from build123d import *

# Parameters (mm, degrees)
SKETCH1_R           = 10.5
SKETCH1_R_2         = 8
BOSS_EXTRUDE1_DEPTH = 3


with BuildPart() as part:
    # Sketch1 → Boss-Extrude1 (new body)
    # profile 1 of 4: a face of its own
    with BuildSketch(Plane.XY):
        Circle(SKETCH1_R)
        Circle(SKETCH1_R_2, mode=Mode.SUBTRACT)
    # profile 2 of 4: a face of its own
    with BuildSketch(Plane.XY):
        with BuildLine():
            ThreePointArc((1, 7.937253933), (0, 8), (-1, 7.937253933))
            Line((-1, 7.937253933), (-1, 5.937253933))
            ThreePointArc((-1, 5.937253933), (0, 6.020879028), (1, 5.937253933))
            Line((1, 5.937253933), (1, 7.937253933))
        make_face()
    # profile 3 of 4: a face of its own
    with BuildSketch(Plane.XY):
        with BuildLine():
            ThreePointArc((6.373863542, -4.83465237), (6.92820323, -4), (7.373863542, -3.102601563))
            Line((7.373863542, -3.102601563), (5.641812735, -2.102601563))
            ThreePointArc((5.641812735, -2.102601563), (5.214234191, -3.010439514), (4.641812735, -3.83465237))
            Line((4.641812735, -3.83465237), (6.373863542, -4.83465237))
        make_face()
    # profile 4 of 4: a face of its own
    with BuildSketch(Plane.XY):
        with BuildLine():
            Line((-5.641812735, -2.102601563), (-7.373863542, -3.102601563))
            ThreePointArc((-7.373863542, -3.102601563), (-6.92820323, -4), (-6.373863542, -4.83465237))
            Line((-6.373863542, -4.83465237), (-4.641812735, -3.83465237))
            ThreePointArc((-4.641812735, -3.83465237), (-5.214234191, -3.010439514), (-5.641812735, -2.102601563))
        make_face()
    extrude(amount=BOSS_EXTRUDE1_DEPTH)


solid = part.part
Verification items for the finished model (mm, model axes). A direction names the side the tool comes from. Give positions to 0.01 mm unless a question says otherwise; leave off trailing zeros. Write each loop counter-clockwise with the first axis right and the second up, starting at its lowest first coordinate (ties: lowest second). Pieces come first, ordered by that corner, then holes. Notation, with made-up numbers: M 31.5,87.25 L 65.5,87.25 A13 ccw 65.5,103.25 Z; hole C 33.5,14 d1. An arc over 180 degrees is marked long. Write item = value, one per line.
(1) Sectioned sample at D-D (x = 9). Record the cut outline in (y, z).
Found:
outline = M -5.41,0 L 5.41,0 L 5.41,3 L -5.41,3 Z
(2) Sectioned sample at B-B (x = 0). Record the cut outline in (y, z).
Found:
outline = M -10.5,0 L -8,0 L -8,3 L -10.5,3 Z; M 6.02,0 L 10.5,0 L 10.5,3 L 6.02,3 Z
(3) Material ranges on line 1 (X direction, y = 0.25, z = 0.7); line 2 (X direction, y = 6.75, z = 2.4); line 3 (Y direction, x = -6.25, z = 1.85), recorded low to high.
Found:
line_1 = -10.5 to -8, 8 to 10.5
line_2 = -8.04 to -4.29, -1 to 1, 4.29 to 8.04
line_3 = -8.44 to -4.99, -4.76 to -2.45, 4.99 to 8.44
(4) Sectioned sample at A-A (y = 0). Record the cut outline in (x, z).
Found:
outline = M -10.5,0 L -8,0 L -8,3 L -10.5,3 Z; M 8,0 L 10.5,0 L 10.5,3 L 8,3 Z
(5) Go/stop test with flat-tipped pins: pin 1 Ø2 at (x, y) = (4, 4.5) entering from +Z; pin 2 Ø1 at (y, z) = (-3.5, 1.5) entering from +X; pin 3 Ø1.5 at (x, z) = (-2.5, 2) entering from -Y; pin 4 Ø0.6 at (y, z) = (6.5, 2) entering from +X. Record where each tip stops, or that it passes through.
Found:
pin_1 = through
pin_2 = 10.06
pin_3 = -10.35
pin_4 = 8.47
(6) Access from +Z, -Z, +X, -X, +Y, -Y to the whole of each face (thin tool, end or side, straight path). Record for faces 5 (the face through (6.5, -2.6, 1.5)), 6 (the face through (0, 6.3, 0)).
Found:
face_5 = +Z, -Z
face_6 = -Z, +X, -X, +Y, -Y
(7) Draft check along Y on faces 1 (the face through (10, 3.2, 1.5)), 2 (the face through (-6.5, -2.6, 1.5)), 3 (the face through (6.98, 3.91, 1.48)), 4 (the face through (0, 6.3, 3)). Enter one of: released by +Y, released by -Y, zero draft, split by the parting line, or undercut.
Found:
face_1 = split by the parting line
face_2 = undercut
face_3 = undercut
face_4 = zero draft
(8) Sectioned sample at C-C (z = 0.95). Record the cut outline in (x, y).
Found:
outline = C 0,0 d21; hole M -7.37,-3.1 L -5.64,-2.1 A6.02 ccw -4.64,-3.83 L -6.37,-4.83 A8 ccw 6.37,-4.83 L 4.64,-3.83 A6.02 ccw 5.64,-2.1 L 7.37,-3.1 A8 ccw 1,7.94 L 1,5.94 A6.02 ccw -1,5.94 L -1,7.94 A8 ccw Z
